Source: CAD feature listing. Evaluate the final solid. Frame: model axes, mm. Coordinates: 2 decimals unless noted, no trailing zeros. Loops run counter-clockwise (first coordinate to the right, second up) from the corner with the lowest first, then second, coordinate; pieces in that order, holes last. Notation, with made-up numbers: M -23.75,-7 L 11.25,-7 A17 ccw 11.25,26 Z; hole C 49.5,38 d11. An arc over 180 degrees is marked long. Write each question's results on one line, items separated by ' | '. Start each with the question number.
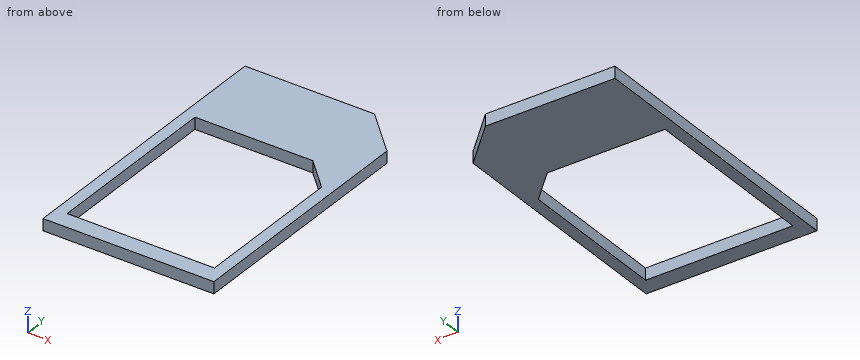
from build123d import *

# Parameters (mm, degrees)
F1_DEPTH = 1


with BuildPart() as f1:
    # F0 (on Top) → F1 (new body)
    with BuildSketch(Plane.XY):
        Polygon((-7.25, -12.25), (7.25, -12.25), (7.25, 8.75), (3.75, 12.25), (-7.25, 12.25), align=None)
        Polygon((6.25, 2.25), (6.25, -10.75), (-6.25, -10.75), (-6.25, 4.75), (3.75, 4.75), align=None, mode=Mode.SUBTRACT)
    extrude(amount=F1_DEPTH)


solid = f1.part
Item 1: Cut plane B-B (y = -6.5). Output: boundary loops of the cut face in (x, z).
Item 2: Cut plane C-C (x = -3.25). Output: boundary loops of the cut face in (y, z).
Item 3: Cut plane A-A (z = 0.25). Output: boundary loops of the cut face in (x, y).
Item 4: Cut plane D-D (y = 10.5). Output: boundary loops of the cut face in (x, z).
Item 5: Line query: probe 1 along Y at (x, z) = (-1.25, 0.9); probe 2 along X at (y, z) = (0.75, 0.85); probe 3 along Y at (x, z) = (4.75, 0.55). Output: solid intervals per line, ascending.
Item 6: First-contact query: pin 1 Ø8 at (x, y) = (0, -2.5) entering from +Z. Flat tip, straight axial feed; report the tip coordinate or a pass-through.
Response values:
1) outline: M -7.25,0 L -6.25,0 L -6.25,1 L -7.25,1 Z; M 6.25,0 L 7.25,0 L 7.25,1 L 6.25,1 Z
2) outline: M -12.25,0 L -10.75,0 L -10.75,1 L -12.25,1 Z; M 4.75,0 L 12.25,0 L 12.25,1 L 4.75,1 Z
3) outline: M -7.25,-12.25 L 7.25,-12.25 L 7.25,8.75 L 3.75,12.25 L -7.25,12.25 Z; hole M -6.25,-10.75 L 6.25,-10.75 L 6.25,2.25 L 3.75,4.75 L -6.25,4.75 Z
4) outline: M -7.25,0 L 5.5,0 L 5.5,1 L -7.25,1 Z
5) probe 1: y = -12.25 to -10.75, 4.75 to 12.25 | probe 2: x = -7.25 to -6.25, 6.25 to 7.25 | probe 3: y = -12.25 to -10.75, 3.75 to 11.25
6) pin 1: passes through
